```python
from build123d import *

# Parameters (mm, degrees)
SALIENTE_EXTRUIR1_DEPTH = 3
CORTAR_EXTRUIR1_REACH   = 5
CROQUIS2_W              = 15.3
CROQUIS2_H              = 3
CROQUIS2_W_2            = 16.15
CROQUIS2_W_3            = 3
CROQUIS2_H_2            = 44.7


with BuildPart() as part:
    # Croquis1 → Saliente-Extruir1 (new body)
    with BuildSketch(Plane.XY):
        with BuildLine():
            Line((101.5, 195), (104.8, 195))
            ThreePointArc((104.8, 195), (105.860660172, 195.439339828), (106.3, 196.5))
            Line((106.3, 196.5), (106.3, 208.5))
            ThreePointArc((106.3, 208.5), (106.739339828, 209.560660172), (107.8, 210))
            Line((107.8, 210), (112.8, 210))
            ThreePointArc((112.8, 210), (113.860660172, 209.560660172), (114.3, 208.5))
            Line((114.3, 208.5), (114.3, 171.5))
            ThreePointArc((114.3, 171.5), (113.860660172, 170.439339828), (112.8, 170))
            Line((112.8, 170), (101.5, 170))
            ThreePointArc((101.5, 170), (100.439339828, 169.560660172), (100, 168.5))
            Line((100, 168.5), (100, 96.5))
            ThreePointArc((100, 96.5), (100.439339828, 95.439339828), (101.5, 95))
            Line((101.5, 95), (104.8, 95))
            ThreePointArc((104.8, 95), (105.860660172, 95.439339828), (106.3, 96.5))
            Line((106.3, 96.5), (106.3, 108.5))
            ThreePointArc((106.3, 108.5), (106.739339828, 109.560660172), (107.8, 110))
            Line((107.8, 110), (112.8, 110))
            ThreePointArc((112.8, 110), (113.860660172, 109.560660172), (114.3, 108.5))
            Line((114.3, 108.5), (114.3, 71.5))
            ThreePointArc((114.3, 71.5), (113.860660172, 70.439339828), (112.8, 70))
            Line((112.8, 70), (101.5, 70))
            ThreePointArc((101.5, 70), (100.439339828, 69.560660172), (100, 68.5))
            Line((100, 68.5), (100, -53.5))
            ThreePointArc((100, -53.5), (100.439339828, -54.560660172), (101.5, -55))
            Line((101.5, -55), (104.8, -55))
            ThreePointArc((104.8, -55), (105.860660172, -54.560660172), (106.3, -53.5))
            Line((106.3, -53.5), (106.3, -41.5))
            ThreePointArc((106.3, -41.5), (106.739339828, -40.439339828), (107.8, -40))
            Line((107.8, -40), (112.8, -40))
            ThreePointArc((112.8, -40), (113.860660172, -40.439339828), (114.3, -41.5))
            Line((114.3, -41.5), (114.3, -78.5))
            ThreePointArc((114.3, -78.5), (113.860660172, -79.560660172), (112.8, -80))
            Line((112.8, -80), (101.5, -80))
            ThreePointArc((101.5, -80), (100.439339828, -80.439339828), (100, -81.5))
            Line((100, -81.5), (100, -153.5))
            ThreePointArc((100, -153.5), (100.439339828, -154.560660172), (101.5, -155))
            Line((101.5, -155), (104.8, -155))
            ThreePointArc((104.8, -155), (105.860660172, -154.560660172), (106.3, -153.5))
            Line((106.3, -153.5), (106.3, -141.5))
            ThreePointArc((106.3, -141.5), (106.739339828, -140.439339828), (107.8, -140))
            Line((107.8, -140), (112.8, -140))
            ThreePointArc((112.8, -140), (113.860660172, -140.439339828), (114.3, -141.5))
            Line((114.3, -141.5), (114.3, -178.5))
            ThreePointArc((114.3, -178.5), (113.860660172, -179.560660172), (112.8, -180))
            Line((112.8, -180), (101.5, -180))
            ThreePointArc((101.5, -180), (100.439339828, -180.439339828), (100, -181.5))
            Line((100, -181.5), (100, -250))
            Line((100, -250), (-100, -250))
            Line((-100, -250), (-100, 250))
            Line((-100, 250), (100, 250))
            Line((100, 250), (100, 196.5))
            ThreePointArc((100, 196.5), (100.439339828, 195.439339828), (101.5, 195))
        make_face()
    extrude(amount=SALIENTE_EXTRUIR1_DEPTH)

    # Croquis2 → Cortar-Extruir1 (cut, up to next)
    with BuildSketch(Plane.XY.offset(3), mode=Mode.PRIVATE) as cortar_extruir1_sk1:
        Polygon((-100, -250), (-80.85, -250), (-80.85, -247), (-97, -247), (-97, -202.65), (-100, -202.65), align=None)
    cortar_extruir1_tool1 = extrude(cortar_extruir1_sk1.sketch, amount=-CORTAR_EXTRUIR1_REACH, mode=Mode.PRIVATE) & part.part
    add(cortar_extruir1_tool1.solids().sort_by_distance((-99.489241, -226.325, 3))[0], mode=Mode.SUBTRACT)
    # Croquis2 → Cortar-Extruir1 (cut, up to next)
    with BuildSketch(Plane.XY.offset(3), mode=Mode.PRIVATE) as cortar_extruir1_sk2:
        with Locations((-43.5, -248.5)):
            Rectangle(CROQUIS2_W, CROQUIS2_H)
    cortar_extruir1_tool2 = extrude(cortar_extruir1_sk2.sketch, amount=-CORTAR_EXTRUIR1_REACH, mode=Mode.PRIVATE) & part.part
    add(cortar_extruir1_tool2.solids().sort_by_distance((-43.5, -248.5, 3))[0], mode=Mode.SUBTRACT)
    # Croquis2 → Cortar-Extruir1 (cut, up to next)
    with BuildSketch(Plane.XY.offset(3), mode=Mode.PRIVATE) as cortar_extruir1_sk3:
        with Locations((1.5, -248.5)):
            Rectangle(CROQUIS2_W, CROQUIS2_H)
    cortar_extruir1_tool3 = extrude(cortar_extruir1_sk3.sketch, amount=-CORTAR_EXTRUIR1_REACH, mode=Mode.PRIVATE) & part.part
    add(cortar_extruir1_tool3.solids().sort_by_distance((1.5, -248.5, 3))[0], mode=Mode.SUBTRACT)
    # Croquis2 → Cortar-Extruir1 (cut, up to next)
    with BuildSketch(Plane.XY.offset(3), mode=Mode.PRIVATE) as cortar_extruir1_sk4:
        with Locations((46.5, -248.5)):
            Rectangle(CROQUIS2_W, CROQUIS2_H)
    cortar_extruir1_tool4 = extrude(cortar_extruir1_sk4.sketch, amount=-CORTAR_EXTRUIR1_REACH, mode=Mode.PRIVATE) & part.part
    add(cortar_extruir1_tool4.solids().sort_by_distance((46.5, -248.5, 3))[0], mode=Mode.SUBTRACT)
    # Croquis2 → Cortar-Extruir1 (cut, up to next)
    with BuildSketch(Plane.XY.offset(3), mode=Mode.PRIVATE) as cortar_extruir1_sk5:
        with Locations((91.925, -248.5)):
            Rectangle(CROQUIS2_W_2, CROQUIS2_H)
    cortar_extruir1_tool5 = extrude(cortar_extruir1_sk5.sketch, amount=-CORTAR_EXTRUIR1_REACH, mode=Mode.PRIVATE) & part.part
    add(cortar_extruir1_tool5.solids().sort_by_distance((91.925, -248.5, 3))[0], mode=Mode.SUBTRACT)
    # Croquis2 → Cortar-Extruir1 (cut, up to next)
    with BuildSketch(Plane.XY.offset(3), mode=Mode.PRIVATE) as cortar_extruir1_sk6:
        with Locations((-98.5, -135)):
            Rectangle(CROQUIS2_W_3, CROQUIS2_H_2)
    cortar_extruir1_tool6 = extrude(cortar_extruir1_sk6.sketch, amount=-CORTAR_EXTRUIR1_REACH, mode=Mode.PRIVATE) & part.part
    add(cortar_extruir1_tool6.solids().sort_by_distance((-98.5, -135, 3))[0], mode=Mode.SUBTRACT)
    # Croquis2 → Cortar-Extruir1 (cut, up to next)
    with BuildSketch(Plane.XY.offset(3), mode=Mode.PRIVATE) as cortar_extruir1_sk7:
        with Locations((-98.5, -45)):
            Rectangle(CROQUIS2_W_3, CROQUIS2_H_2)
    cortar_extruir1_tool7 = extrude(cortar_extruir1_sk7.sketch, amount=-CORTAR_EXTRUIR1_REACH, mode=Mode.PRIVATE) & part.part
    add(cortar_extruir1_tool7.solids().sort_by_distance((-98.5, -45, 3))[0], mode=Mode.SUBTRACT)
    # Croquis2 → Cortar-Extruir1 (cut, up to next)
    with BuildSketch(Plane.XY.offset(3), mode=Mode.PRIVATE) as cortar_extruir1_sk8:
        with Locations((-98.5, 45)):
            Rectangle(CROQUIS2_W_3, CROQUIS2_H_2)
    cortar_extruir1_tool8 = extrude(cortar_extruir1_sk8.sketch, amount=-CORTAR_EXTRUIR1_REACH, mode=Mode.PRIVATE) & part.part
    add(cortar_extruir1_tool8.solids().sort_by_distance((-98.5, 45, 3))[0], mode=Mode.SUBTRACT)
    # Croquis2 → Cortar-Extruir1 (cut, up to next)
    with BuildSketch(Plane.XY.offset(3), mode=Mode.PRIVATE) as cortar_extruir1_sk9:
        with Locations((-98.5, 135)):
            Rectangle(CROQUIS2_W_3, CROQUIS2_H_2)
    cortar_extruir1_tool9 = extrude(cortar_extruir1_sk9.sketch, amount=-CORTAR_EXTRUIR1_REACH, mode=Mode.PRIVATE) & part.part
    add(cortar_extruir1_tool9.solids().sort_by_distance((-98.5, 135, 3))[0], mode=Mode.SUBTRACT)
    # Croquis2 → Cortar-Extruir1 (cut, up to next)
    with BuildSketch(Plane.XY.offset(3), mode=Mode.PRIVATE) as cortar_extruir1_sk10:
        Polygon((-80.85, 247), (-80.85, 250), (-100, 250), (-100, 202.65), (-97, 202.65), (-97, 247), align=None)
    cortar_extruir1_tool10 = extrude(cortar_extruir1_sk10.sketch, amount=-CORTAR_EXTRUIR1_REACH, mode=Mode.PRIVATE) & part.part
    add(cortar_extruir1_tool10.solids().sort_by_distance((-81.360759, 248.5, 3))[0], mode=Mode.SUBTRACT)
    # Croquis2 → Cortar-Extruir1 (cut, up to next)
    with BuildSketch(Plane.XY.offset(3), mode=Mode.PRIVATE) as cortar_extruir1_sk11:
        with Locations((-43.5, 248.5)):
            Rectangle(CROQUIS2_W, CROQUIS2_H)
    cortar_extruir1_tool11 = extrude(cortar_extruir1_sk11.sketch, amount=-CORTAR_EXTRUIR1_REACH, mode=Mode.PRIVATE) & part.part
    add(cortar_extruir1_tool11.solids().sort_by_distance((-43.5, 248.5, 3))[0], mode=Mode.SUBTRACT)
    # Croquis2 → Cortar-Extruir1 (cut, up to next)
    with BuildSketch(Plane.XY.offset(3), mode=Mode.PRIVATE) as cortar_extruir1_sk12:
        with BuildLine():
            ThreePointArc((41.5, 155), (59.17766953, 162.32233047), (66.5, 180))
            ThreePointArc((66.5, 180), (59.17766953, 197.67766953), (41.5, 205))
            Line((41.5, 205), (-38.5, 205))
            ThreePointArc((-38.5, 205), (-63.5, 180), (-38.5, 155))
            Line((-38.5, 155), (41.5, 155))
        make_face()
    cortar_extruir1_tool12 = extrude(cortar_extruir1_sk12.sketch, amount=-CORTAR_EXTRUIR1_REACH, mode=Mode.PRIVATE) & part.part
    add(cortar_extruir1_tool12.solids().sort_by_distance((1.5, 180, 3))[0], mode=Mode.SUBTRACT)
    # Croquis2 → Cortar-Extruir1 (cut, up to next)
    with BuildSketch(Plane.XY.offset(3), mode=Mode.PRIVATE) as cortar_extruir1_sk13:
        with Locations((46.5, 248.5)):
            Rectangle(CROQUIS2_W, CROQUIS2_H)
    cortar_extruir1_tool13 = extrude(cortar_extruir1_sk13.sketch, amount=-CORTAR_EXTRUIR1_REACH, mode=Mode.PRIVATE) & part.part
    add(cortar_extruir1_tool13.solids().sort_by_distance((46.5, 248.5, 3))[0], mode=Mode.SUBTRACT)
    # Croquis2 → Cortar-Extruir1 (cut, up to next)
    with BuildSketch(Plane.XY.offset(3), mode=Mode.PRIVATE) as cortar_extruir1_sk14:
        with Locations((1.5, 248.5)):
            Rectangle(CROQUIS2_W, CROQUIS2_H)
    cortar_extruir1_tool14 = extrude(cortar_extruir1_sk14.sketch, amount=-CORTAR_EXTRUIR1_REACH, mode=Mode.PRIVATE) & part.part
    add(cortar_extruir1_tool14.solids().sort_by_distance((1.5, 248.5, 3))[0], mode=Mode.SUBTRACT)
    # Croquis2 → Cortar-Extruir1 (cut, up to next)
    with BuildSketch(Plane.XY.offset(3), mode=Mode.PRIVATE) as cortar_extruir1_sk15:
        with Locations((91.925, 248.5)):
            Rectangle(CROQUIS2_W_2, CROQUIS2_H)
    cortar_extruir1_tool15 = extrude(cortar_extruir1_sk15.sketch, amount=-CORTAR_EXTRUIR1_REACH, mode=Mode.PRIVATE) & part.part
    add(cortar_extruir1_tool15.solids().sort_by_distance((91.925, 248.5, 3))[0], mode=Mode.SUBTRACT)
    # Croquis2 → Cortar-Extruir1 (cut, up to next)
    with BuildSketch(Plane.XY.offset(3), mode=Mode.PRIVATE) as cortar_extruir1_sk16:
        with BuildLine():
            ThreePointArc((41.5, -205), (59.17766953, -197.67766953), (66.5, -180))
            ThreePointArc((66.5, -180), (59.17766953, -162.32233047), (41.5, -155))
            Line((41.5, -155), (-38.5, -155))
            ThreePointArc((-38.5, -155), (-63.5, -180), (-38.5, -205))
            Line((-38.5, -205), (41.5, -205))
        make_face()
    cortar_extruir1_tool16 = extrude(cortar_extruir1_sk16.sketch, amount=-CORTAR_EXTRUIR1_REACH, mode=Mode.PRIVATE) & part.part
    add(cortar_extruir1_tool16.solids().sort_by_distance((1.5, -180, 3))[0], mode=Mode.SUBTRACT)


solid = part.part
```
Verification items for the finished model (mm, model axes). A direction names the side the tool comes from. Give positions to 0.01 mm unless a question says otherwise; leave off trailing zeros. Order: outer loops, then holes, each group sorted by start corner. A loop starts at its lowest first (then second) coordinate and runs counter-clockwise, first axis right, second up. Notation, with made-up numbers: (56.25, 9.5) - (90.25, 9.5) arc R21 ccw to (90.25, 13.5) - close; hole circle Ø3 at (39, 26). An arc over 180 degrees is marked (long way). Answer as CSV lines item,"result". Start each with the question number.
Item 1: Section check B-B, the plane y = -167. Record the boundary of the cut face in (x, z), plus the area to 3 significant figures.
Item 2: Section check A-A, the plane x = 27.5. Record the boundary of the cut face in (y, z).
Item 3: Section check C-C, the plane z = 2.05. State how many separate pieces and enclosed holes the cut face has, plus the area to 3 significant figures.
Item 4: Section check D-D, the plane y = 44. Record the boundary of the cut face in (x, z).
Item 5: Access from +Z, -Z, +X, -X, +Y, -Y to the whole of each face (thin tool, end or side, straight path). Record for faces 1 (the face through (9, 4, 3)), 2 (the face through (-63.494, -179.45, 1.521)).
Item 6: Gauge pin test, flat ends, axial feed: pin 1 (1.5 mm diameter, centred on y = -248.5, z = 1, fed in from -X); pin 2 (0.9 mm diameter, centred on y = -248.5, z = 1, fed in from +X); pin 3 (0.9 mm diameter, centred on y = -40.5, z = 2, fed in from -X). Record the tip position at first contact, or that the pin passes through.
Item 7: Material ranges on L1, parallel to Y at x = -27, z = 1.35; L2, parallel to Y at x = 4, z = 2.5; L3, parallel to X at y = 106.5, z = 0.65, recorded low to high.
Item 8: Mould release check, pull along Y, two halves, no side actions. Record for faces 3 (the face through (9, 4, 0)), 4 (the face through (-63.494, 180.55, 1.521)): released by +Y, released by -Y, zero draft, split by the parting line, or undercut.
Filled in:
1,outline,"(-100, 0) - (-59.85, 0) - (-59.85, 3) - (-100, 3) - close; (62.85, 0) - (114.3, 0) - (114.3, 3) - (62.85, 3) - close"
1,area,"275 mm^2"
2,outline,"(-250, 0) - (-205, 0) - (-205, 3) - (-250, 3) - close; (-155, 0) - (155, 0) - (155, 3) - (-155, 3) - close; (205, 0) - (250, 0) - (250, 3) - (205, 3) - close"
3,separate pieces,"1"
3,enclosed holes,"2"
3,area,"88,700 mm^2"
4,outline,"(-97, 0) - (100, 0) - (100, 3) - (-97, 3) - close"
5,face 1,"+Z, +X, -X, +Y, -Y"
5,face 2,"+Z, -Z"
6,pin 1,"x = -80.85"
6,pin 2,"x = 83.85"
6,pin 3,"x = -97"
7,L1,"-250 to -205, -155 to 155, 205 to 250"
7,L2,"-247 to -205, -155 to 155, 205 to 247"
7,L3,"-100 to 100, 106.3 to 114.3"
8,face 3,"zero draft"
8,face 4,"undercut"
